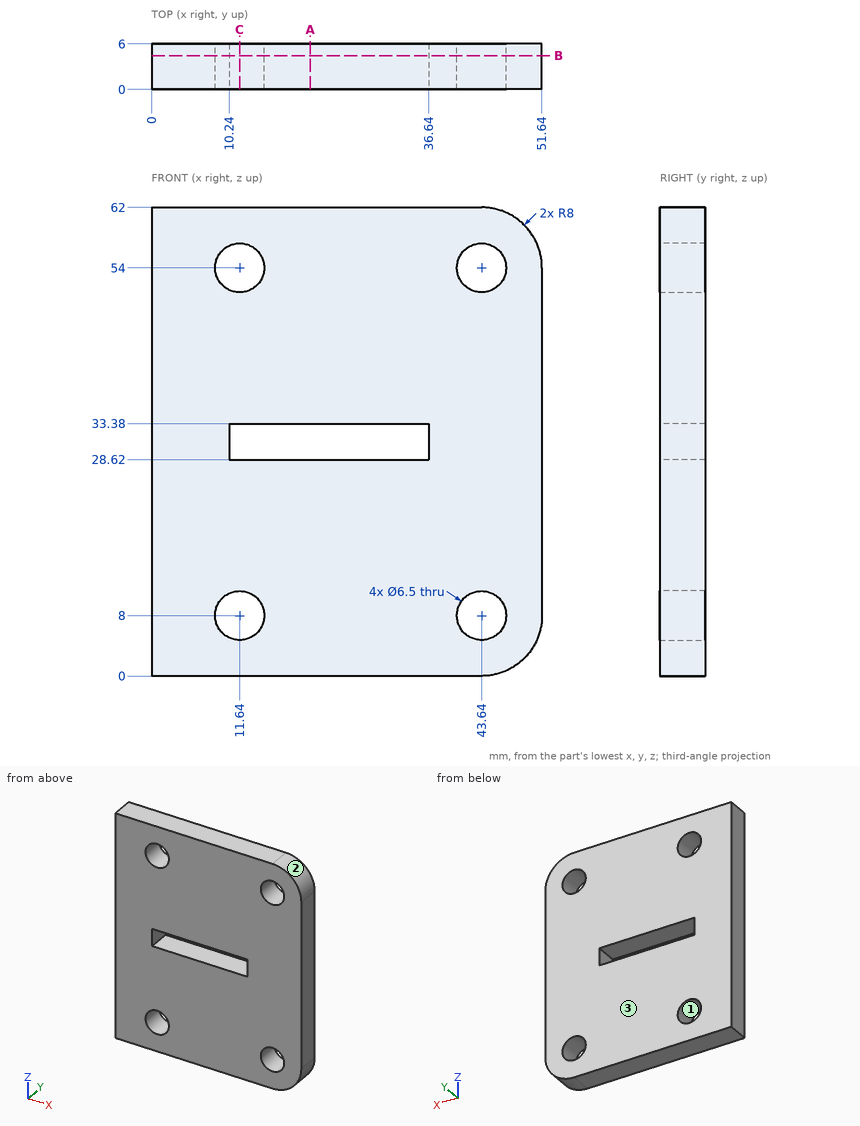
Can you work these out from the drawing? Everything is in mm from the part's minimum corner. Round coordinates to 2 decimals unless told otherwise and drop trailing zeros. Loops run counter-clockwise (first coordinate to the right, second up) from the corner with the lowest first, then second, coordinate; pieces in that order, holes last. Notation, with made-up numbers: M 17.25,23 L 58.25,23 A14 cw 58.25,49 Z; hole C -26.5,7 d6. An arc over 180 degrees is marked long. Write item = value, one per line.
1. Thinking about a two-plate mould opening in X: for the marked faces 1, 2 and 3, which applies, +X half, -X half, draft (parallel to the pull), parting line (faces both ways), or undercut?
Results below:
face_1 = undercut
face_2 = +X half
face_3 = draft
2. I need wall thicknesses on probe 1 along X at (y, z) = (1.5, 8); probe 2 along Z at (x, y) = (31, 4.7); probe 3 along X at (y, z) = (4.35, 53). Which ranges of each line are inside material? Lowest first, please.
Results below:
probe_1 = 0 to 8.39, 14.89 to 40.39, 46.89 to 51.64
probe_2 = 0 to 28.62, 33.38 to 62
probe_3 = 0 to 8.55, 14.73 to 40.55, 46.73 to 51.64
3. I want a section at A-A, the plane x = 21. Write out the boundary of the cut face in (y, z).
Results below:
outline = M 0,0 L 6,0 L 6,28.62 L 0,28.62 Z; M 0,33.38 L 6,33.38 L 6,62 L 0,62 Z
4. I want a section at B-B, the plane y = 4.45. Write out the boundary of the cut face in (x, z), and give its area (3 significant figures).
Results below:
outline = M 0,0 L 43.64,0 A8 ccw 51.64,8 L 51.64,54 A8 ccw 43.64,62 L 0,62 Z; hole C 11.64,8 d6.5; hole C 11.64,54 d6.5; hole M 10.24,28.62 L 36.64,28.62 L 36.64,33.38 L 10.24,33.38 Z; hole C 43.64,8 d6.5; hole C 43.64,54 d6.5
area = 2,920 mm²
5. I want a section at C-C, the plane x = 11.64. Write out the boundary of the cut face in (y, z), and give its area (3 significant figures).
Results below:
outline = M 0,0 L 6,0 L 6,4.75 L 0,4.75 Z; M 0,11.25 L 6,11.25 L 6,28.62 L 0,28.62 Z; M 0,33.38 L 6,33.38 L 6,50.75 L 0,50.75 Z; M 0,57.25 L 6,57.25 L 6,62 L 0,62 Z
area = 265 mm²
